Geometry check sheet. Reference: the model listing, model coordinates, mm. Face numbers are marked on the shaded views. A direction names the side the tool comes from. Coordinates: 2 decimals unless noted, no trailing zeros. Order: outer loops, then holes, each group sorted by start corner. A loop starts at its lowest first (then second) coordinate and runs counter-clockwise, first axis right, second up. Notation, with made-up numbers: (-2.5, 89.5) - (25.5, 89.5) arc R20 ccw to (25.5, 97.5) - close; hole circle Ø10 at (33, 87.5). An arc over 180 degrees is marked (long way). Return JSON: item names as keys, results as strings. Group by question number.
Item 1: Section check C-C on z = -1.2. Enter the section's corners in (x, y), then the cut area to 3 significant figures.
Item 2: Section check A-A on y = 6. Give the number of separate pieces and of enclosed holes in the cut face, then the cut area to 3 significant figures.
Item 3: Draft check along X on the marked faces 3, 4 and 5. Enter one of: pulls with the +X half, pulls with the -X half, needs draft (parallel to the pull), parting line crosses it, or undercut.
Item 4: Tool access check on the marked faces 1 and 2. Record the directions out of +Z, -Z, +X, -X, +Y, -Y that give a thin tool (end or side, any length) a straight path to the whole face; none if there is none.
Item 5: Scan lines: probe 1 along X at (y, z) = (5.5, -1.75); probe 2 along Z at (x, y) = (6.5, 4.25); probe 3 along Y at (x, z) = (-3.25, 1.7). Record each from-to range of solid material in increasing order.
Item 6: Section check D-D on x = -4.75. Enter the section's corners in (y, z).
Item 7: Gauge pin test, flat ends, axial feed: pin 1 (1 mm diameter, centred on x = -4.5, z = 0.5, fed in from -Y); pin 2 (5 mm diameter, centred on x = 1, y = 5.5, fed in from -Z) (3 decimals). Record the tip position at first contact, or that the pin passes through.
Autodesk Inventor part; units mm, degrees
ref_plane "YZ Plane" through (0, 0, 0) normal (1, 0, 0) x (0, 1, 0)
ref_plane "XZ Plane" through (0, 0, 0) normal (0, 1, 0) x (-1, 0, 0)
ref_plane "XY Plane" through (0, 0, 0) normal (0, 0, 1) x (1, 0, 0)
sketch "Sketch1" plane through (0, 0, 0) normal (0, 1, 0) x (-1, 0, 0)
  line L0 (-7.5, -2.5) -> (7.5, -2.5)
  line L1 (7.5, -2.5) -> (7.5, 2.5)
  line L2 (7.5, 2.5) -> (-7.5, 2.5)
  line L3 (-7.5, 2.5) -> (-7.5, -2.5)
  line L4 (-7.5, -2.5) -> (7.5, 2.5) construction
  line L5 (7.5, -2.5) -> (-7.5, 2.5) construction
  point P0 (0, 0)
  dimension "d0" = 15
  dimension "d1" = 5
extrude "Extrusion1" add sketch "Sketch1" along normal blind 1
sketch "Sketch2" plane through (0, 1, 0) normal (0, 1, 0) x (1, 0, 0)
  line L0 (7.5, 2.5) -> (-7.5, 2.5)
  line L1 (-7.5, 2.5) -> (-7.5, -2.5)
  line L2 (-7.5, -2.5) -> (7.5, -2.5)
  line L3 (7.5, -2.5) -> (7.5, 2.5)
  line L4 (-5.1536, 2.5) -> (-5.1536, 2.2)
  line L5 (-5.1536, 2.2) -> (-7.2, 2.2)
  line L6 (-7.2, 2.2) -> (-7.2, -2.2)
  line L7 (-7.2, -2.2) -> (0, -2.2)
  line L8 (0, -2.2) -> (0, -2.5)
  line L9 (7.5, 2.5) -> (-7.5, 2.5)
  line L10 (-5.1536, 2.5) -> (-7.5, 2.5)
  line L11 (-7.5, 2.5) -> (-7.5, -2.5)
  point P0 (0, 0)
  dimension "d4" = 0.3
  dimension "d5" = 0.3
  dimension "d6" = 0.3
extrude "Extrusion2" add sketch "Sketch2" along normal blind 6 contours L4 L5 L6 L7 L8 L2 L1 L0
mirror "Mirror1" about plane through (0, 0, 0) normal (1, 0, 0) of "Extrusion2"
sketch "Sketch3" plane through (7.5, 0, -2.5) normal (0, 0, -1) x (-1, 0, 0)
  line L0 (0, 0) -> (15, 0)
  line L1 (15, 0) -> (15, 7)
  line L2 (12.6536, 7) -> (15, 7)
  line L3 (12.6536, 1) -> (12.6536, 7)
  line L4 (2.3464, 1) -> (12.6536, 1)
  line L5 (2.3464, 1) -> (2.3464, 7)
  line L6 (2.3464, 7) -> (0, 7)
  line L7 (0, 0) -> (0, 7)
  line L8 (14.5, 1.5) -> (13.25, 1.5)
  line L9 (13.25, 1.5) -> (13.25, 4)
  line L10 (13.25, 4) -> (14.5, 4)
  line L11 (14.5, 4) -> (14.5, 1.5)
  line L12 (14.5, 1.5) -> (13.25, 4) construction
  line L13 (13.25, 1.5) -> (14.5, 4) construction
  point P0 (7.5, 0)
  point P1 (13.875, 2.75)
  dimension "d9" = 1.25
  dimension "d10" = 2.5
  dimension "d11" = 0.5
  dimension "d12" = 0.5
extrude "Extrusion3" cut sketch "Sketch3" against normal up to surface (0.3 mm away) contours L8 L9 L10 L11
mirror "Mirror2" about plane through (0, 0, 0) normal (1, 0, 0) of "Extrusion3"
sketch "Sketch4" plane through (0, 1, 0) normal (0, 1, 0) x (1, 0, 0)
  line L0 (0, 0) -> (-21.8742, 0)
  circle A0 centre (-5.1429, 0.5) radius 0.125
  line L1 (7.2, -2.2) -> (7.2, 2.2)
  line L2 (-7.2, -2.2) -> (-7.2, 2.2)
  dimension "d15" = 0.25
  dimension "d16" = 0.5
  dimension "d17" = 14.4
  dimension "d18" = 2.0571
extrude "Extrusion4" add sketch "Sketch4" along normal blind 5.25 and the other way blind 2.625
pattern_linear "Rectangular Pattern1" count 6 spacing 2.0571 along (1, 0, 0) of "Extrusion4"
sketch "Sketch5" plane through (-7.5, 0, -2.5) normal (-1, 0, 0) x (0, 0, 1)
  line L0 (0, 0) -> (5, 0)
  line L1 (5, 0) -> (5, 7)
  line L2 (0, 7) -> (5, 7)
  line L3 (0, 0) -> (0, 7)
  line L4 (1, 7) -> (2, 7)
  line L5 (2, 7) -> (2, 5)
  line L6 (2, 5) -> (1, 5)
  line L7 (1, 5) -> (1, 7)
  point P0 (2.5, 0)
  dimension "d26" = 1
  dimension "d27" = 2
  dimension "d28" = 1
extrude "Extrusion5" cut sketch "Sketch5" against normal up to surface (0.3 mm away) contours L2 L5 L6 L7
mirror "Mirror3" about plane through (0, 0, 0) normal (1, 0, 0) of "Extrusion5"
equation "\"d5\" = d4"
equation "\"d6\" = d5"
equation "\"d12\" = d11"
equation "\"d18\" = 0.142857 * d17"
equation "\"d23\" = 0.142857 * d17"
equation "\"d28\" = d26"
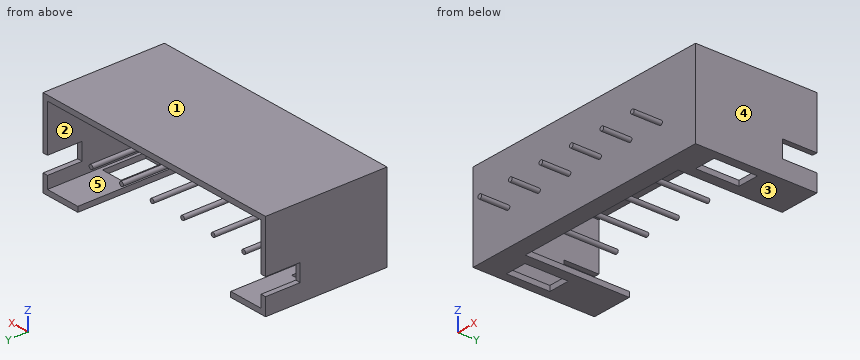
Computed:
{
 "1": {"outline": "(-7.5, 0) - (7.5, 0) - (7.5, 5) - (7.2, 5) - (7.2, 1) - (-7.2, 1) - (-7.2, 5) - (-7.5, 5) - close", "area": "17.4 mm²"},
 "2": {"separate pieces": "9", "enclosed holes": "0", "area": "8.24 mm²"},
 "3": {"face 3": "needs draft", "face 4": "pulls with the +X half", "face 5": "undercut"},
 "4": {"face 1": "+Z, +X, -X, +Y, -Y", "face 2": "+Y"},
 "5": {"probe 1": "x = -7.5 to -7.2, 7.2 to 7.5", "probe 2": "z = -2.5 to -2.2, 2.2 to 2.5", "probe 3": "y = 0 to 1"},
 "6": {"outline": "(0, -2.5) - (1, -2.5) - (1, 2.2) - (7, 2.2) - (7, 2.5) - (0, 2.5) - close"},
 "7": {"pin 1": "stops at y = 0", "pin 2": "stops at z = -0.625"}
}
